Drawing for the job (mm, zero at the part's lowest x, y, z). A direction names the side the tool comes from. Coordinates: 2 decimals unless noted, no trailing zeros. Write each loop counter-clockwise with the first axis right and the second up, starting at its lowest first coordinate (ties: lowest second). Pieces come first, ordered by that corner, then holes. Notation, with made-up numbers: (43.5, 59.25) - (101.5, 59.25) arc R14 cw to (101.5, 72.25) - close; hole circle Ø8 at (-30, -20). An arc over 180 degrees is marked (long way). Write each question's results on one line, items separated by ' | '.
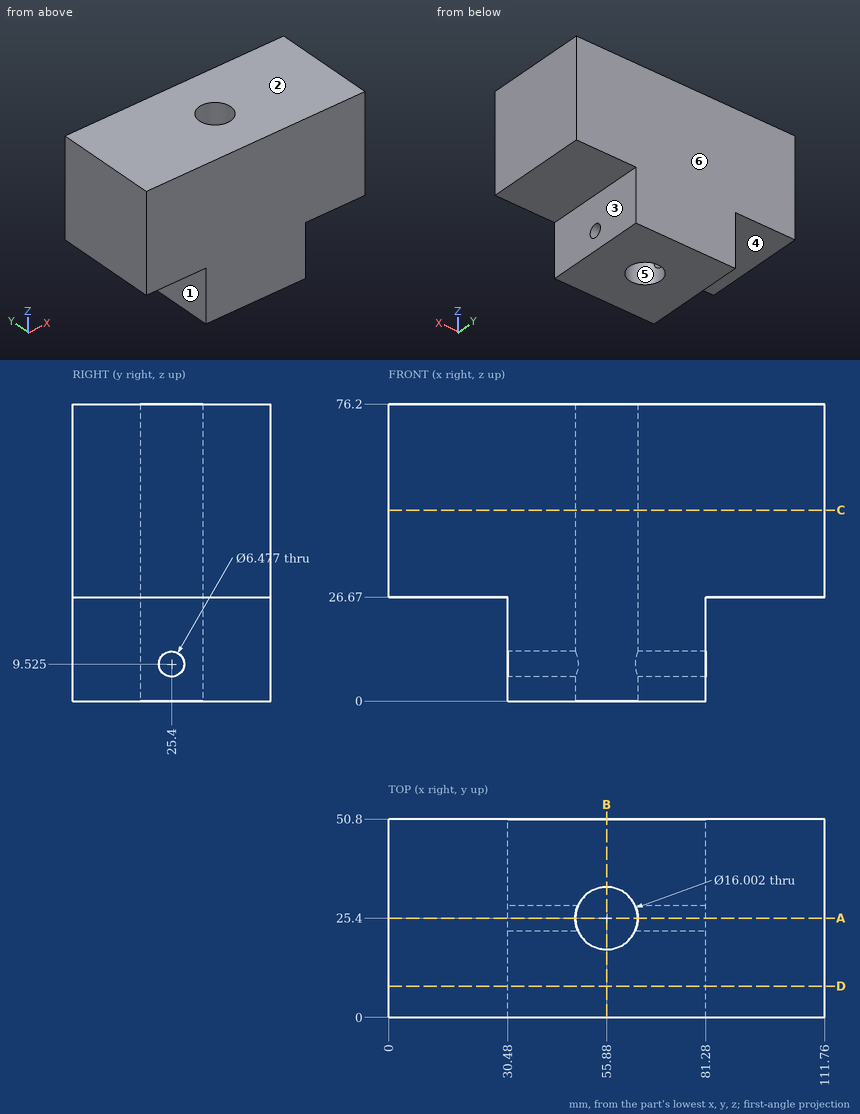
(1) Flat gauge pins, fed straight in: P1, Ø1, axis at x = 82, y = 37, coming from the -Z side; P2, Ø9.5, axis at x = 55.88, y = 25.4, coming from the -Z side; P3, Ø4, axis at y = 29, z = 19.5, coming from the -X side; P4, Ø10.5, axis at y = 25.4, z = 9.525, coming from the +X side. Where does each tip first touch, or does it go through?
Return value:
P1: stops at z = 26.67 | P2: passes through | P3: stops at x = 30.48 | P4: stops at x = 81.28
(2) Saw through at D-D on y = 8. Write the cut outline in (x, z).
Return value:
outline: (0, 26.67) - (30.48, 26.67) - (30.48, 0) - (81.28, 0) - (81.28, 26.67) - (111.76, 26.67) - (111.76, 76.2) - (0, 76.2) - close
(3) 3-axis set-ups, long thin cutter, end or side, ignore diameter. For the marked faces 1, 2 and 3: which of +Z, -Z, +X, -X, +Y, -Y reach the whole face in a straight line?
Return value:
face 1: -Z, -X, +Y, -Y | face 2: +Z, +X, -X, +Y, -Y | face 3: -Z, +X, +Y, -Y
(4) Two-plate mould, pull along Y, no slides. Class the marked faces 4, 5 and 6: released by +Y, released by -Y, zero draft, split by the parting line, or undercut.
Return value:
face 4: zero draft | face 5: undercut | face 6: released by +Y
(5) Saw through at C-C on z = 49. Write the cut outline in (x, y), then the cut area to 3 significant figures.
Return value:
outline: (0, 0) - (111.76, 0) - (111.76, 50.8) - (0, 50.8) - close; hole circle Ø16 at (55.88, 25.4) | area: 5,480 mm^2
(6) Wall check: line 1 (Z direction, x = 38.75, y = 25.4); line 2 (X direction, y = 25, z = 55); line 3 (Z direction, x = 11.5, y = 15). Give the ranges that are in metal, low to high. Write a range as from..to.
Return value:
line 1: z = 0..6.29, 12.76..76.2 | line 2: x = 0..47.89, 63.87..111.76 | line 3: z = 26.67..76.2
(7) Saw through at A-A on y = 25.4. Write the cut outline in (x, z), then the cut area to 3 significant figures.
Return value:
outline: (0, 26.67) - (30.48, 26.67) - (30.48, 12.76) - (47.88, 12.76) - (47.88, 76.2) - (0, 76.2) - close; (30.48, 0) - (47.88, 0) - (47.88, 6.29) - (30.48, 6.29) - close; (63.88, 0) - (81.28, 0) - (81.28, 6.29) - (63.88, 6.29) - close; (63.88, 12.76) - (81.28, 12.76) - (81.28, 26.67) - (111.76, 26.67) - (111.76, 76.2) - (63.88, 76.2) - close | area: 5,450 mm^2
(8) Saw through at B-B on x = 55.88. Write the cut outline in (y, z).
Return value:
outline: (0, 0) - (17.4, 0) - (17.4, 76.2) - (0, 76.2) - close; (33.4, 0) - (50.8, 0) - (50.8, 76.2) - (33.4, 76.2) - close
